from build123d import *

# Parameters (mm, degrees)
BOSS_EXTRUDE1_DEPTH = 4.5
CUT_EXTRUDE1_DEPTH  = 2.5


with BuildPart() as part:
    # Sketch1 → Boss-Extrude1 (new body)
    with BuildSketch(Plane(origin=(0, 0, 0), x_dir=(1, 0, 0), z_dir=(0, 1, 0))):
        with BuildLine():
            Line((-13, 0), (-9.43, 0))
            ThreePointArc((-9.43, 0), (0, 9.43), (9.43, 0))
            Line((9.43, 0), (13, 0))
            ThreePointArc((13, 0), (0, 13), (-13, 0))
        make_face()
    extrude(amount=BOSS_EXTRUDE1_DEPTH)

    # Sketch2 → Cut-Extrude1 (cut)
    with BuildSketch(Plane(origin=(0, 4.5, 0), x_dir=(1, 0, 0), z_dir=(0, 1, 0))):
        with BuildLine():
            Line((-13, 0), (-11.43, 0))
            ThreePointArc((-11.43, 0), (0, 11.43), (11.43, 0))
            Line((11.43, 0), (13, 0))
            ThreePointArc((13, 0), (0, 13), (-13, 0))
        make_face()
    extrude(amount=-CUT_EXTRUDE1_DEPTH, mode=Mode.SUBTRACT)


solid = part.part
Could you check a few things on this model? Use its own coordinates, in mm. A direction names the side the tool comes from. Coordinates: 2 decimals unless noted, no trailing zeros. Order: outer loops, then holes, each group sorted by start corner. A loop starts at its lowest first (then second) coordinate and runs counter-clockwise, first axis right, second up.
Q1. Which directions (+Z, -Z, +X, -X, +Y, -Y) give clear straight access to the entire face, cutting with the end or side of a thin tool? Please do faces 1 (the flat face through (-11, 2, 0)), 2 (the cylindrical face through (-0.251, 3.268, -11.427)).
Q2. Suppose I cut it at A-A on x = 0. Please give me the cut outline in (y, z), and give its area (3 significant figures).
Q3. Suppose I cut it at C-C on y = 0.45. Please give me the cut outline in (x, z).
Q4. Suppose I cut it at D-D on z = -11. Please give me the cut outline in (x, y).
Q5. Thinking about a two-plate mould opening in X: for faces 3 (the flat face through (11, 2, 0)), 4 (the cylindrical face through (-0.207, 2.218, -9.428)), 5 (the cylindrical face through (0, 1, -13)), which applies, released by +X, released by -X, zero draft, split by the parting line, or undercut?
Q6. Please list where these lines run through material, in increasing order: L1, parallel to X at y = 3.4, z = -2.5; L2, parallel to Y at x = 2.75, z = -12; L3, parallel to X at y = 3.9, z = -7.
Q7. Will these pins go through, and if not, where does the flat tip stop? pin 1 (6 mm diameter, centred on x = -2.5, z = -2.5, fed in from -Y); pin 2 (1 mm diameter, centred on x = 4, y = 2, fed in from +Z); pin 3 (1.5 mm diameter, centred on y = 3, z = -8.5, fed in from +X).
Q8. Suppose I cut it at B-B on z = -6.5. Please give me the cut outline in (x, y), and give its area (3 significant figures).
Answer:
1. face 1: +Z, +X, -X, +Y, -Y
1. face 2: -Z, +Y
2. outline: (0, -13) - (2, -13) - (2, -11.43) - (4.5, -11.43) - (4.5, -9.43) - (0, -9.43) - close
2. area: 12.1 mm2
3. outline: (-13, 0) arc R13 ccw to (13, 0) - (9.43, 0) arc R9.43 cw to (-9.43, 0) - close
4. outline: (-6.93, 0) - (6.93, 0) - (6.93, 2) - (3.11, 2) - (3.11, 4.5) - (-3.11, 4.5) - (-3.11, 2) - (-6.93, 2) - close
5. face 3: zero draft
5. face 4: undercut
5. face 5: split by the parting line
6. L1: x = -11.15 to -9.09, 9.09 to 11.15
6. L2: y = 0 to 2
6. L3: x = -9.04 to -6.32, 6.32 to 9.04
7. pin 1: passes through
7. pin 2: stops at z = -8.29
7. pin 3: stops at x = 8.4
8. outline: (-11.26, 0) - (-6.83, 0) - (-6.83, 4.5) - (-9.4, 4.5) - (-9.4, 2) - (-11.26, 2) - close; (6.83, 0) - (11.26, 0) - (11.26, 2) - (9.4, 2) - (9.4, 4.5) - (6.83, 4.5) - close
8. area: 30.6 mm2
